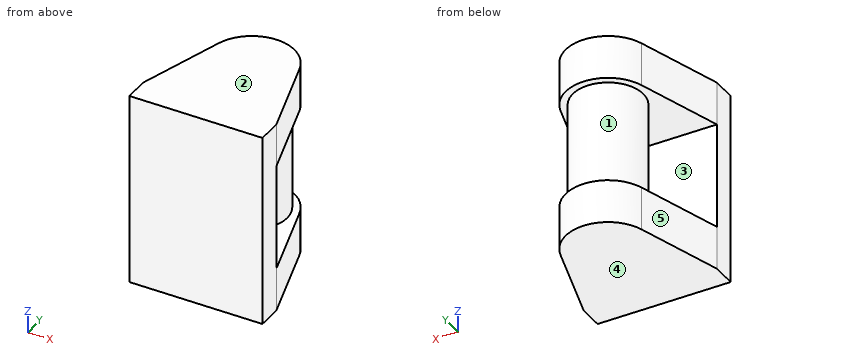
from build123d import *

# Parameters (mm, degrees)
F0_W     = 2.75
F0_H     = 1
F0_R     = 1.45
F1_DEPTH = 1.8
F2_DEPTH = 4


# Not quite as in the source:
# - a feature of the source that left no trace in its solid (it failed there, or was rolled back) is left out


with BuildPart() as f1:
    # F0 (on Top) → F1 (new body)
    with BuildSketch(Plane.XY):
        with Locations((1.375, 0.5)):
            Rectangle(F0_W, F0_H)
        with Locations((-1.375, 0.5)):
            Rectangle(F0_W, F0_H)
        with BuildLine():
            Line((0, 2.3), (0, 1))
            Line((0, 1), (2.75, 1))
            Line((2.75, 1), (1.675161779, 4.5562934073))
            ThreePointArc((1.675161779, 4.5562934073), (1.7311893474, 4.3058973298), (1.75, 4.05))
            ThreePointArc((1.75, 4.05), (1.2374368671, 2.8125631329), (0, 2.3))
        make_face()
        with BuildLine():
            Line((-2.75, 1), (0, 1))
            Line((0, 1), (0, 2.3))
            ThreePointArc((0, 2.3), (-1.4050824643, 3.0068110101), (-1.675161779, 4.5562934073))
            Line((-1.675161779, 4.5562934073), (-2.75, 1))
        make_face()
        with BuildLine():
            ThreePointArc((-1.675161779, 4.5562934073), (-1.4050824643, 3.0068110101), (0, 2.3))
            ThreePointArc((0, 2.3), (1.2374368671, 2.8125631329), (1.75, 4.05))
            ThreePointArc((1.75, 4.05), (1.7311893474, 4.3058973298), (1.675161779, 4.5562934073))
            ThreePointArc((1.675161779, 4.5562934073), (0, 5.8), (-1.675161779, 4.5562934073))
        make_face()
        with Locations((0, 4.05)):
            Circle(F0_R, mode=Mode.SUBTRACT)
        with Locations((0, 4.05)):
            Circle(F0_R)
    extrude(amount=F1_DEPTH)

    # F0 (on Top) → F2 (join)
    with BuildSketch(Plane.XY):
        with Locations((0, 4.05)):
            Circle(F0_R)
        with Locations((-1.375, 0.5)):
            Rectangle(F0_W, F0_H)
        with Locations((1.375, 0.5)):
            Rectangle(F0_W, F0_H)
    extrude(amount=F2_DEPTH)

    # F4: F1 across plane


with BuildPart() as f1_1:
    add(f1.part)
    add(f1.part.mirror(Plane.XY.offset(4)))


solid = f1_1.part
Verification items for the finished model (mm, model axes). Face numbers are marked on the shaded views. A direction names the side the tool comes from. Round coordinates to 2 decimals unless told otherwise and drop trailing zeros. Order: outer loops, then holes, each group sorted by start corner. A loop starts at its lowest first (then second) coordinate and runs counter-clockwise, first axis right, second up.
1. Section check A-A on x = 0. Record the cut outline in (y, z), then the cut area to 3 significant figures.
Final values:
outline: (0, 0) - (5.8, 0) - (5.8, 1.8) - (5.5, 1.8) - (5.5, 6.2) - (5.8, 6.2) - (5.8, 8) - (0, 8) - close; hole (1, 1.8) - (2.6, 1.8) - (2.6, 6.2) - (1, 6.2) - close
area: 38.0 mm2
2. Access from +Z, -Z, +X, -X, +Y, -Y to the whole of each face (thin tool, end or side, straight path). Record for the marked faces 1 and 2.
Final values:
face 1: none
face 2: +Z, +X, -X, +Y, -Y
3. Release check for a two-part mould opening along Y. For the marked faces 3, 4 and 5 record: +Y half, -Y half, draft (parallel to the pull), parting line (faces both ways), or undercut.
Final values:
face 3: undercut
face 4: draft
face 5: +Y half
4. Section check D-D on z = 1.25. Record the cut outline in (x, y).
Final values:
outline: (-2.75, 0) - (2.75, 0) - (2.75, 1) - (1.68, 4.56) arc R1.75 ccw to (-1.68, 4.56) - (-2.75, 1) - close
5. Thickness scan on L1, parallel to Y at x = 0.05, z = 5.25; L2, parallel to Z at x = 1.55, y = 4.8; L3, parallel to Y at x = 1.85, z = 2. Record the ranges inside material, lowest first.
Final values:
L1: y = 0 to 1, 2.6 to 5.5
L2: z = 0 to 1.8, 6.2 to 8
L3: y = 0 to 1
6. Section check B-B on z = 2.75. Record the cut outline in (x, y), then the cut area to 3 significant figures.
Final values:
outline: (-2.75, 0) - (2.75, 0) - (2.75, 1) - (-2.75, 1) - close; circle Ø2.9 at (0, 4.05)
area: 12.1 mm2
7. Section check C-C on y = 5.1. Record the cut outline in (x, z).
Final values:
outline: (-1.4, 0) - (1.4, 0) - (1.4, 1.8) - (1, 1.8) - (1, 6.2) - (1.4, 6.2) - (1.4, 8) - (-1.4, 8) - (-1.4, 6.2) - (-1, 6.2) - (-1, 1.8) - (-1.4, 1.8) - close
8. Go/stop test with a flat-tipped pin: P1, Ø1.3, axis at x = -1, z = 4, coming from the +Y side. Record where the tip stops, or that it passes through.
Final values:
P1: stops at y = 5.46
